```python
from build123d import *

# Parameters (mm, degrees)
F1_DEPTH = 2.9718
F2_R     = 1.651
F2_R_2   = 2.159
F2_R_3   = 0.889
F3_DEPTH = 25.4


with BuildPart() as f1:
    # F0 (on Top) → F1 (new body)
    with BuildSketch(Plane.XY):
        Polygon((0, 69.85), (0, 0), (12.7, 0), (12.7, 16.383), (17.78, 16.383), (17.78, 22.733), (12.7, 22.733), (12.7, 47.117), (17.78, 47.117), (17.78, 53.467), (12.7, 53.467), (12.7, 69.85), align=None)
    extrude(amount=F1_DEPTH)

    # F2 (on face) → F3 (cut)
    with BuildSketch(Plane.XY.offset(2.9718)):
        with Locations((14.1986, 50.292)):
            Circle(F2_R)
        with Locations((14.1986, 19.558)):
            Circle(F2_R)
        with Locations((6.35, 34.925)):
            Circle(F2_R_2)
        with Locations((6.35, 39.116)):
            Circle(F2_R_3)
        with Locations((6.35, 30.734)):
            Circle(F2_R_3)
    extrude(amount=-F3_DEPTH, mode=Mode.SUBTRACT)


solid = f1.part
```
For this review, take the finished solid that the model builds, in its own axes (mm). A direction names the side the tool comes from. Round coordinates to 2 decimals unless told otherwise and drop trailing zeros. Loops run counter-clockwise (first coordinate to the right, second up) from the corner with the lowest first, then second, coordinate; pieces in that order, holes last.
Q1. Add section C-C on y = 15. Write out the cut boundary in (x, z).
Result sheet:
outline: (0, 0) - (12.7, 0) - (12.7, 2.97) - (0, 2.97) - close
Q2. Machinability: for faces 1 (the face through (15, 47.117, 1)), 2 (the face through (12.7, 62, 1)), 3 (the face through (15, 16.383, 1)), which of the approach directions +Z, -Z, +X, -X, +Y, -Y give a long, thin tool a straight path to every point of the face, cutting with its end or side? Answer none if there is none.
Result sheet:
face 1: +Z, -Z, +X
face 2: +Z, -Z, +X, +Y
face 3: +Z, -Z, +X, -Y
Q3. Insertion check: pin 1 Ø0.9 at (x, z) = (15, 2) entering from +Y; pin 2 Ø1.5 at (y, z) = (11, 2) entering from +X; pin 3 Ø0.9 at (x, z) = (14.5, 1.5) entering from -Y; pin 4 Ø4 at (x, y) = (6.35, 34.925) entering from -Z. Each pin has a flat end and moves straight along its axis. Give the tip position at first contact, or say it passes through.
Result sheet:
pin 1: stops at y = 53.47
pin 2: stops at x = 12.7
pin 3: stops at y = 16.38
pin 4: passes through
Q4. Mouldability with a two-part tool opening along Y and no side actions: class faces 4 (the face through (13.84, 48.68, 1.51)), 5 (the face through (6, 0, 1)), 6 (the face through (17.78, 50, 1)) as +Y half, -Y half, draft (parallel to the pull), parting line (faces both ways), or undercut.
Result sheet:
face 4: undercut
face 5: -Y half
face 6: draft
Q5. To check wall thickness, follow line 1 along Y through (x, z) = (6.35, 1.1) (3 decimals); line 2 along Y through (x, z) = (16.5, 1.85); line 3 along X through (y, z) = (66.5, 1.3). State the ranges of each line that lie inside material, in increasing order.
Result sheet:
line 1: y = 0 to 29.845, 31.623 to 32.766, 37.084 to 38.227, 40.005 to 69.85
line 2: y = 16.38 to 22.73, 47.12 to 53.47
line 3: x = 0 to 12.7
Q6. Add section A-A on x = 6.35. Write out the cut boundary in (y, z) (3 decimals).
Result sheet:
outline: (0, 0) - (29.845, 0) - (29.845, 2.972) - (0, 2.972) - close; (31.623, 0) - (32.766, 0) - (32.766, 2.972) - (31.623, 2.972) - close; (37.084, 0) - (38.227, 0) - (38.227, 2.972) - (37.084, 2.972) - close; (40.005, 0) - (69.85, 0) - (69.85, 2.972) - (40.005, 2.972) - close
Q7. Add section B-B on z = 1.3. Write out the cut boundary in (x, y) (3 decimals).
Result sheet:
outline: (0, 0) - (12.7, 0) - (12.7, 16.383) - (17.78, 16.383) - (17.78, 22.733) - (12.7, 22.733) - (12.7, 47.117) - (17.78, 47.117) - (17.78, 53.467) - (12.7, 53.467) - (12.7, 69.85) - (0, 69.85) - close; hole circle Ø4.318 at (6.35, 34.925); hole circle Ø1.778 at (6.35, 30.734); hole circle Ø1.778 at (6.35, 39.116); hole circle Ø3.302 at (14.199, 19.558); hole circle Ø3.302 at (14.199, 50.292)
